Input: part model. Units: mm. Frame: model coordinates. Coordinates: 2 decimals unless noted, no trailing zeros. Loops run counter-clockwise (first coordinate to the right, second up) from the corner with the lowest first, then second, coordinate; pieces in that order, holes last. Notation, with made-up numbers: (52, 63.25) - (58, 63.25) arc R10 cw to (58, 82.25) - close; hole circle Ø8 at (-30, -27.75). An arc over 180 degrees is marked (long way). Use a Markdown table: item, result. Add a question column.
1. Section query A-A on x = 0. Return the cut outline in (y, z), then the cut area to 3 significant figures.
2. Section query D-D on x = 10. Return the cut outline in (y, z).
3. Ray query, L1, parallel to X at y = 26, z = 0; L2, parallel to Y at x = 17, z = 9. Return the intervals inside material, ascending. Write a range as [from, to].
4. Contact query for flat-ended pins moving along their axis: P1, Ø10, axis at x = -4.5, z = -16, coming from the -Y side; P2, Ø2, axis at y = 27.5, z = 17.5, coming from the +X side; P3, Ø3, axis at y = 27.5, z = -1, coming from the +X side; P4, Ø2.5, axis at x = 0, z = -10, coming from the +Y side. Output: stop coordinate, or through.
5. Section query B-B on z = -10. Return the cut outline in (x, y).
6. Section query C-C on y = 29.25. Return the cut outline in (x, z).
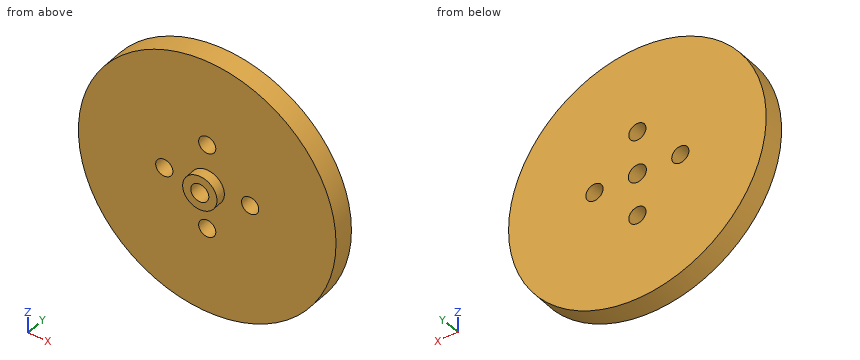
```python
from build123d import *

# Parameters (mm, degrees)
CROQUIS1_R              = 2.05
CROQUIS1_R_2            = 4
SALIENTE_EXTRUIR1_DEPTH = 25.4
CROQUIS2_R              = 30
SALIENTE_EXTRUIR2_DEPTH = 5
CROQUIS3_R              = 2
CORTAR_EXTRUIR1_DEPTH   = 7.5
CROQUIS7_R              = 3.5
CORTAR_EXTRUIR3_DEPTH   = 3
CROQUIS8_W              = 62.698346187
CROQUIS8_H              = 3
CORTAR_EXTRUIR5_DEPTH   = 15
CROQUIS1_3_R            = 2.05
CORTAR_EXTRUIR6_DEPTH   = 7.4
SALIENTE_EXTRUIR3_DEPTH = 10
CROQUIS6_R              = 1.25
CORTAR_EXTRUIR7_DEPTH   = 10
CROQUIS10_R             = 4.00257807
CORTAR_EXTRUIR8_DEPTH   = 20
CROQUIS11_R             = 2.1
CORTAR_EXTRUIR9_DEPTH   = 20


with BuildPart() as part:
    # Croquis1 → Saliente-Extruir1 (new body)
    with BuildSketch(Plane(origin=(0, 0, 0), x_dir=(1, 0, 0), z_dir=(0, 1, 0))):
        Circle(CROQUIS1_R)
        Circle(CROQUIS1_R_2)
        Circle(CROQUIS1_R, mode=Mode.SUBTRACT)
    extrude(amount=SALIENTE_EXTRUIR1_DEPTH)

    # Croquis2 → Saliente-Extruir2 (add)
    with BuildSketch(Plane(origin=(0, 25.4, 0), x_dir=(1, 0, 0), z_dir=(0, 1, 0))):
        Circle(CROQUIS2_R)
    extrude(amount=SALIENTE_EXTRUIR2_DEPTH)

    # Croquis3 → Cortar-Extruir1 (cut)
    with BuildSketch(Plane(origin=(0, 30.4, 0), x_dir=(1, 0, 0), z_dir=(0, 1, 0))):
        with Locations((0, 10)):
            Circle(CROQUIS3_R)
        with Locations((10, 0)):
            Circle(CROQUIS3_R)
        with Locations((0, -10)):
            Circle(CROQUIS3_R)
        with Locations((-10, 0)):
            Circle(CROQUIS3_R)
    extrude(amount=-CORTAR_EXTRUIR1_DEPTH, mode=Mode.SUBTRACT)

    # Croquis7 → Cortar-Extruir3 (cut)
    with BuildSketch(Plane.XZ):
        Circle(CROQUIS7_R)
    extrude(amount=-CORTAR_EXTRUIR3_DEPTH, mode=Mode.SUBTRACT)

    # Croquis8 → Cortar-Extruir5 (cut, symmetric)
    with BuildSketch(Plane(origin=(0, 0, 0), x_dir=(0, 0, -1), z_dir=(1, 0, 0))):
        with Locations((4.276742622, 1.5)):
            Rectangle(CROQUIS8_W, CROQUIS8_H)
    extrude(amount=CORTAR_EXTRUIR5_DEPTH, both=True, mode=Mode.SUBTRACT)

    # Croquis1<3> → Cortar-Extruir6 (cut)
    with BuildSketch(Plane(origin=(0, 0, 0), x_dir=(1, 0, 0), z_dir=(0, 1, 0))):
        Circle(CROQUIS1_3_R)
    extrude(amount=CORTAR_EXTRUIR6_DEPTH, mode=Mode.SUBTRACT)

    # Croquis9 → Saliente-Extruir3 (add)
    with BuildSketch(Plane.XZ.offset(-3)):
        with BuildLine():
            ThreePointArc((1.281600562, 1.6), (0, 2.05), (-1.281600562, 1.6))
            Line((-1.281600562, 1.6), (1.281600562, 1.6))
        make_face()
    extrude(amount=-SALIENTE_EXTRUIR3_DEPTH)

    # Croquis6 → Cortar-Extruir7 (cut)
    with BuildSketch(Plane.XY):
        with Locations((0, 5)):
            Circle(CROQUIS6_R)
    extrude(amount=CORTAR_EXTRUIR7_DEPTH, mode=Mode.SUBTRACT)

    # Croquis10 → Cortar-Extruir8 (cut)
    with BuildSketch(Plane.XZ.offset(-3)):
        Circle(CROQUIS10_R)
    extrude(amount=-CORTAR_EXTRUIR8_DEPTH, mode=Mode.SUBTRACT)

    # Croquis11 → Cortar-Extruir9 (cut)
    with BuildSketch(Plane(origin=(0, 30.4, 0), x_dir=(1, 0, 0), z_dir=(0, 1, 0))):
        Circle(CROQUIS11_R)
    extrude(amount=-CORTAR_EXTRUIR9_DEPTH, mode=Mode.SUBTRACT)


solid = part.part
```
Resolved:
| question | item | result |
|---|---|---|
| 1 | outline | (23, -4) - (25.4, -4) - (25.4, -8) - (30.4, -8) - (30.4, -2.1) - (23, -2.1) - close; (23, 2.1) - (30.4, 2.1) - (30.4, 8) - (25.4, 8) - (25.4, 4) - (23, 4) - close; (25.4, -30) - (30.4, -30) - (30.4, -12) - (25.4, -12) - close; (25.4, 12) - (30.4, 12) - (30.4, 30) - (25.4, 30) - close |
| 1 | area | 248 mm² |
| 2 | outline | (25.4, -28.28) - (30.4, -28.28) - (30.4, -2) - (25.4, -2) - close; (25.4, 2) - (30.4, 2) - (30.4, 28.28) - (25.4, 28.28) - close |
| 3 | L1 | [-30, -12], [-8, -2.1], [2.1, 8], [12, 30] |
| 3 | L2 | [25.4, 30.4] |
| 4 | P1 | y = 25.4 |
| 4 | P2 | x = 25.05 |
| 4 | P3 | x = 30 |
| 4 | P4 | through |
| 5 | outline | (-28.28, 25.4) - (-2, 25.4) - (-2, 30.4) - (-28.28, 30.4) - close; (2, 25.4) - (28.28, 25.4) - (28.28, 30.4) - (2, 30.4) - close |
| 6 | outline | circle Ø60 at (0, 0); hole circle Ø4 at (-10, 0); hole circle Ø4.2 at (0, 0); hole circle Ø4 at (0, -10); hole circle Ø4 at (0, 10); hole circle Ø4 at (10, 0) |
